from build123d import *

# Parameters (mm, degrees)
SKETCH2_W           = 92
SKETCH2_H           = 91.562656452
SKETCH2_R           = 25
BOSS_EXTRUDE1_DEPTH = 3


with BuildPart() as part:
    # Sketch1 → Revolve1 (revolve)
    with BuildSketch(Plane.XY, mode=Mode.PRIVATE) as revolve1_sk:
        Polygon((-27.28653196, 0), (-46, 9.100705487), (-45.562656452, 10), (-25, 0), align=None)
    revolve(revolve1_sk.sketch.rotate(Axis((0, 0, 0), (0, 1, 0)), 270), axis=Axis((0, 0, 0), (0, 1, 0)))



with BuildPart() as body_2:
    # Sketch2 → Boss-Extrude1 (new body)
    with BuildSketch(Plane(origin=(0, 0, 0), x_dir=(1, 0, 0), z_dir=(0, 1, 0))):
        with Locations((0, -0.218671774)):
            Rectangle(SKETCH2_W, SKETCH2_H)
        with Locations(Location((0, -0.218671774, 0), (0, 0, 270))):
            Circle(SKETCH2_R, mode=Mode.SUBTRACT)
    extrude(amount=-BOSS_EXTRUDE1_DEPTH)


with BuildPart() as part_1:
    add(part.part)

    add(body_2.part)  # Revolve2 merges body 2
    # Sketch3 → Revolve2 (revolve)
    with BuildSketch(Plane.XY, mode=Mode.PRIVATE) as revolve2_sk:
        with BuildLine():
            Line((-27.28653196, 0), (-30.485609044, 1.555770331))
            ThreePointArc((-30.485609044, 1.555770331), (-30.045608993, 0.6353225), (-30.843850544, 0))
            Line((-30.843850544, 0), (-27.28653196, 0))
        make_face()
    revolve(revolve2_sk.sketch.rotate(Axis((0, 0, 0), (0, 1, 0)), 270), axis=Axis((0, 0, 0), (0, 1, 0)))


solid = part_1.part
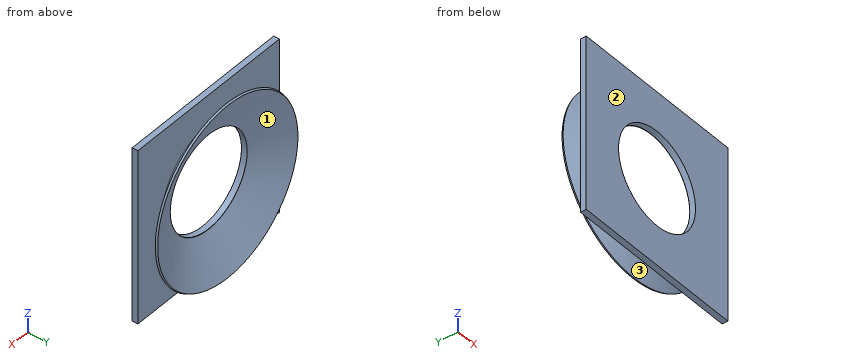
Model file for the job. Use its own axes, mm. Face numbers are marked on the shaded views. Give positions to 0.01 mm unless a question says otherwise; leave off trailing zeros. Order: outer loops, then holes, each group sorted by start corner. A loop starts at its lowest first (then second) coordinate and runs counter-clockwise, first axis right, second up. Notation, with made-up numbers: M 46.5,83.5 L 62.5,83.5 A22 ccw 62.5,101.5 Z; hole C 37.25,-31.75 d2. An arc over 180 degrees is marked long. Put each result on its own line as item: value. Start each with the question number.
(1) Pull direction X, two halves, no side cores. Call the marked faces 1, 2 and 3: released by +X, released by -X, zero draft, split by the parting line, or undercut.
(2) Pin check, flat tips, straight feed: pin 1 Ø8 at (x, z) = (36, -29) entering from +Y; pin 2 Ø1 at (x, y) = (-35.5, -1.5) entering from -Z; pin 3 Ø7.5 at (x, z) = (-10.5, -18.5) entering from +Y; pin 4 Ø6 at (y, z) = (6.5, 13.5) entering from +X. Stop position of each tip, or through.
(3) Band-saw the part on A-A on x = 0. Give the cut face in (y, z), then the cut area to 3 significant figures.
(4) Band-saw the part on B-B on y = 2.75. Give the cut face in (x, z), then the cut area to 3 significant figures.
(5) Drill centre lines: L1, parallel to Z at x = 0, y = -0.7; L2, parallel to Y at x = -41, z = -24; L3, parallel to X at y = 4.75, z = 1. Where is each one in solid material? Low to high. Write a range as [from, to].
Results below:
1. face 1: undercut
1. face 2: zero draft
1. face 3: split by the parting line
2. pin 1: stops at y = 10
2. pin 2: stops at z = -45.56
2. pin 3: stops at y = 0.01
2. pin 4: stops at x = 44.41
3. outline: M -3,-45.56 L 0,-45.56 L 0,-30.84 A0.82 cw 1.56,-30.49 L 9.1,-46 L 10,-45.56 L 0,-25 L 0,-24.78 L -3,-24.78 Z; M -3,25.22 L 0,25.22 L 0,25 L 10,45.56 L 9.1,46 L 1.56,30.49 A0.82 cw 0,30.84 L 0,46 L -3,46 Z
3. area: 172 mm2
4. outline: C 0,0 d65.88; hole C 0,0 d61.31
4. area: 457 mm2
5. L1: z = [-45.56, -24.78], [25.22, 46]
5. L2: y = [-3, 0]
5. L3: x = [-37.04, -34.75], [34.75, 37.04]
